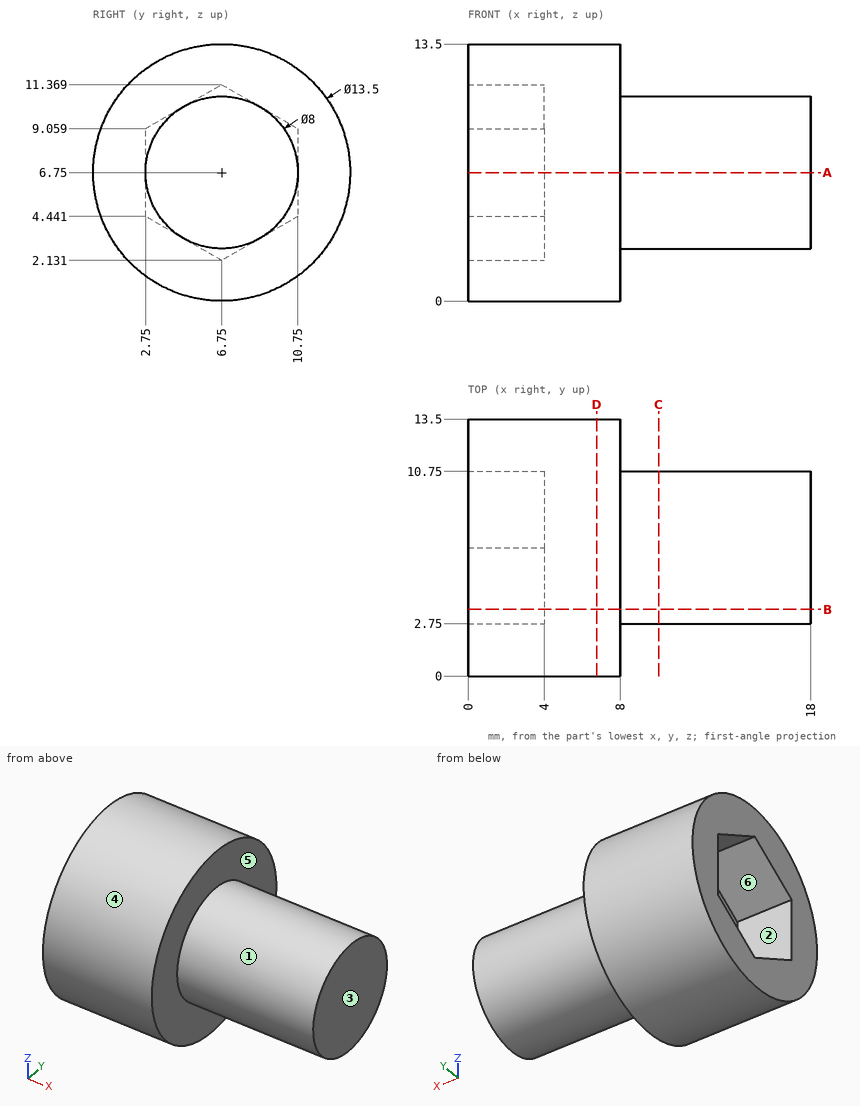
Here's the drawing with two shaded views (mm, measured from the low corner). I have some questions. A direction names the side the tool comes from. Give positions to 0.01 mm unless a question says otherwise; leave off trailing zeros. Loops run counter-clockwise (first coordinate to the right, second up) from the corner with the lowest first, then second, coordinate; pieces in that order, holes last. Notation, with made-up numbers: M 42,-24.75 L 71,-24.75 A30 cw 71,-1.75 Z; hole C -34.75,10.5 d6. An arc over 180 degrees is marked long. One line per item, written item: value. Start each with the question number.
1) If we section it at C-C, the plane x = 10: Write out the boundary of the cut face in (y, z).
2) On a 3-axis mill with a long thin cutter (end or side, diameter ignored), from which of +Z, -Z, +X, -X, +Y, -Y can I reach the whole of each face in a straight line? I mean the marked faces 4, 5 and 6. Say none if no direction works.
3) If we section it at B-B, the plane y = 3.5: Write out the boundary of the cut face in (x, z), and give its area (3 significant figures).
4) If we section it at A-A, the plane z = 6.75: Write out the boundary of the cut face in (x, y).
5) If we section it at D-D, the plane x = 6.75: Write out the boundary of the cut face in (y, z), and give its area (3 significant figures).
6) If I drill on line 1 (X direction, y = 9.25, z = 2.25); line 2 (Z direction, x = 2.25, y = 7.5) (1 decimal); line 3 (X direction, y = 8.5, z = 10.25), over which ranges is the centre line in solid material (lowest first)? Write a range as [from, to].
7) Thinking about a two-plate mould opening in Y: for the marked faces 1, 2 and 3, which applies, +Y half, -Y half, draft (parallel to the pull), parting line (faces both ways), or undercut?
8) I'm going to push flat-ended pins straight in: pin 1 (1 mm diameter, centred on x = 16, y = 3.5, fed in from -Z) (1 decimal); pin 2 (4 mm diameter, centred on y = 8, z = 5.5, fed in from -X); pin 3 (1.5 mm diameter, centred on x = 10, z = 3, fed in from +Y) (1 decimal). Where does each tip first touch, or does it pass through?
Completed:
1. outline: C 6.75,6.75 d8
2. face 4: +X, -X
2. face 5: +X
2. face 6: -X
3. outline: M 0,0.83 L 8,0.83 L 8,4.42 L 18,4.42 L 18,9.08 L 8,9.08 L 8,12.67 L 0,12.67 L 0,9.49 L 4,9.49 L 4,4.01 L 0,4.01 Z
3. area: 119 mm^2
4. outline: M 0,0 L 8,0 L 8,2.75 L 18,2.75 L 18,10.75 L 8,10.75 L 8,13.5 L 0,13.5 L 0,10.75 L 4,10.75 L 4,2.75 L 0,2.75 Z
5. outline: C 6.75,6.75 d13.5
5. area: 143 mm^2
6. line 1: x = [0, 8]
6. line 2: z = [0, 2.6], [10.9, 13.5]
6. line 3: x = [4, 18]
7. face 1: parting line
7. face 2: undercut
7. face 3: draft
8. pin 1: stops at z = 3.8
8. pin 2: stops at x = 4
8. pin 3: stops at y = 9.4
